```python
from build123d import *

# Parameters (mm, degrees)
NECK_DEPTH = 10.9982


# Read off the part's stored shape, not the designer's step: Cut-Revolve1
with BuildPart() as part:
    # Cut-Revolve1 outline → Cut-Revolve1 (revolve)
    with BuildSketch(Plane.YX):
        Polygon((0, 38.1), (0, 0), (11.6586, 0), (11.6586, 0.550820297), (4.7625, 5.0292), (4.7625, 38.1), align=None)
    revolve(axis=Axis((0, 0, 0), (1, 0, 0)))

    # Sketch2 → Neck (add)
    with BuildSketch(Plane(origin=(0, 0, 0), x_dir=(0, 0.6946583704589985, -0.7193398003386501), z_dir=(1, 0, 0))):
        with BuildLine():
            Line((3.6068, -4.8006), (-3.6068, -4.8006))
            ThreePointArc((-3.6068, -4.8006), (-4.450944075, -4.450944075), (-4.8006, -3.6068))
            Line((-4.8006, -3.6068), (-4.8006, 3.6068))
            ThreePointArc((-4.8006, 3.6068), (-4.450944075, 4.450944075), (-3.6068, 4.8006))
            Line((-3.6068, 4.8006), (3.6068, 4.8006))
            ThreePointArc((3.6068, 4.8006), (4.450944075, 4.450944075), (4.8006, 3.6068))
            Line((4.8006, 3.6068), (4.8006, -3.6068))
            ThreePointArc((4.8006, -3.6068), (4.450944075, -4.450944075), (3.6068, -4.8006))
        make_face()
    extrude(amount=NECK_DEPTH)


solid = part.part
```
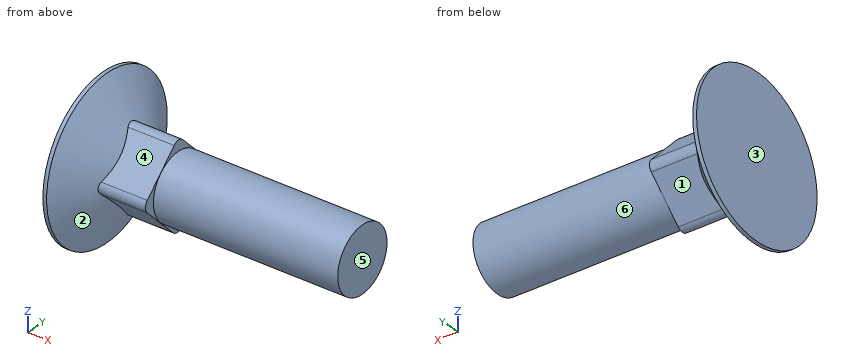
Can you work these out from the model? Positions are in its coordinate system, mm. Face numbers are marked on the shaded views. A direction names the side the tool comes from. Give positions to 0.01 mm unless a question says otherwise; leave off trailing zeros. Order: outer loops, then holes, each group sorted by start corner. A loop starts at its lowest first (then second) coordinate and runs counter-clockwise, first axis right, second up. Notation, with made-up numbers: M 11,-13.5 L 41,-13.5 A29 ccw 41,16.5 Z; hole C 1,-0.75 d4. An arc over 180 degrees is marked long. Write item = value, one per line. Start each with the question number.
Q1. For the marked faces 4, 5 and 6, which set-ups out of +Z, -Z, +X, -X, +Y, -Y let a thin tool reach every point of the face, with its end or its side?
Q2. We'd pull the mould along Z, two halves only. Please class the marked faces 1, 2 and 3: pulls with the +Z half, pulls with the -Z half, needs draft (parallel to the pull), parting line crosses it, or undercut.
Q3. Suppose I cut it at A-A (x = 7). Write out the boundary of the cut face in (y, z), plus the area to 3 significant figures.
Q4. Suppose I cut it at B-B (y = 0). Write out the boundary of the cut face in (x, z), plus the area to 3 significant figures.
Q5. Will these pins go through, and if not, where does the flat tip stop? pin 1 Ø8 at (x, y) = (12, 8.5) entering from +Z; pin 2 Ø10 at (x, z) = (16, -9) entering from -Y; pin 3 Ø5 at (x, y) = (25.5, 5.5) entering from -Z.
Q6. Suppose I cut it at D-D (x = 25.5). Write out the boundary of the cut face in (y, z) (1 decimal).
Q7. I need wall thicknesses on probe 1 along Z at (x, y) = (25, 0); probe 2 along Z at (x, y) = (22, -4); probe 3 along X at (y, z) = (9.25, 6). Which ranges of each line are inside material? Lowest first, please. Write a range as [from, to].
Check result:
q1.face_4 = +Z, +X, -Y
q1.face_5 = +Z, -Z, +X, +Y, -Y
q1.face_6 = +X
q2.face_1 = pulls with the -Z half
q2.face_2 = parting line crosses it
q2.face_3 = needs draft
q3.outline = M -5.96,-0.74 L -0.95,-5.93 A1.19 ccw 0.74,-5.96 L 5.93,-0.95 A1.19 ccw 5.96,0.74 L 0.95,5.93 A1.19 ccw -0.74,5.96 L -5.93,0.95 A1.19 ccw Z
q3.area = 91.0 mm2
q4.outline = M 0,-11.66 L 0.55,-11.66 L 4.04,-6.29 L 11,-6.29 L 11,-4.76 L 38.1,-4.76 L 38.1,4.76 L 11,4.76 L 11,6.29 L 4.04,6.29 L 0.55,11.66 L 0,11.66 Z
q4.area = 421 mm2
q5.pin_1 = 2.12
q5.pin_2 = -2.58
q5.pin_3 = -3.7
q6.outline = C 0,0 d9.5
q7.probe_1 = [-4.76, 4.76]
q7.probe_2 = [-2.58, 2.58]
q7.probe_3 = [0, 0.96]
